from build123d import *

# Parameters (mm, degrees)
ESBO_O1_W                = 93
ESBO_O1_H                = 50
RESSALTO_EXTRUS_O1_DEPTH = 1.26
ESBO_O2_W                = 93
ESBO_O2_H                = 1.26
RESSALTO_EXTRUS_O2_DEPTH = 32.74
ESBO_O3_W                = 1.26
ESBO_O3_H                = 50
RESSALTO_EXTRUS_O4_DEPTH = 32.74
RESSALTO_EXTRUS_O5_START = 25
RESSALTO_EXTRUS_O5_DEPTH = 67
FILETE1_R                = 1
FILETE2_R                = 1
ESBO_O6_W                = 1.26
ESBO_O6_H                = 50
RESSALTO_EXTRUS_O6_DEPTH = 31.48
ESBO_O7_W                = 11
ESBO_O7_H                = 2.5
CORTE_EXTRUS_O1_DEPTH    = 1.26
ESBO_O8_W                = 13
ESBO_O8_H                = 2.5
CORTE_EXTRUS_O2_DEPTH    = 1.26
RESSALTO_EXTRUS_O7_DEPTH = 2
RESSALTO_EXTRUS_O8_DEPTH = 2
ESBO_O13_R               = 0.5
RESSALTO_EXTRUS_O9_DEPTH = 4


with BuildPart() as part:
    # Esboço1 → Ressalto-extrusão1 (new body)
    with BuildSketch(Plane(origin=(0, 0, 0), x_dir=(1, 0, 0), z_dir=(0, 1, 0))):
        with Locations((46.5, -25)):
            Rectangle(ESBO_O1_W, ESBO_O1_H)
    extrude(amount=RESSALTO_EXTRUS_O1_DEPTH)

    # Esboço2 → Ressalto-extrusão2 (add)
    with BuildSketch(Plane(origin=(0, 0, 0), x_dir=(1, 0, 0), z_dir=(0, 1, 0))):
        with Locations((46.5, -0.63)):
            Rectangle(ESBO_O2_W, ESBO_O2_H)
        with Locations((46.5, -49.37)):
            Rectangle(ESBO_O2_W, ESBO_O2_H)
    extrude(amount=RESSALTO_EXTRUS_O2_DEPTH)

    # Esboço3 → Ressalto-extrusão4 (add)
    with BuildSketch(Plane(origin=(0, 0, 0), x_dir=(1, 0, 0), z_dir=(0, 1, 0))):
        with Locations((92.37, -25)):
            Rectangle(ESBO_O3_W, ESBO_O3_H)
    extrude(amount=RESSALTO_EXTRUS_O4_DEPTH)

    # Esboço5 → Ressalto-extrusão5 (add)
    with BuildSketch(Plane(origin=(0, 0, 0), x_dir=(0, 0, -1), z_dir=(1, 0, 0)).offset(RESSALTO_EXTRUS_O5_START)):
        Polygon((0, 32.74), (-3.26, 32.74), (0, 29.48), align=None)
        Polygon((-50, 32.74), (-46.74, 32.74), (-50, 29.48), align=None)
    extrude(amount=RESSALTO_EXTRUS_O5_DEPTH)

    # Filete1
    filete1_edges = [part.edges().sort_by_distance(p)[0] for p in [
        (25, 31.74, 47.74),
    ]]
    fillet(filete1_edges, radius=FILETE1_R)

    # Filete2
    filete2_edges = [part.edges().sort_by_distance(p)[0] for p in [
        (25, 31.74, 2.26),
    ]]
    fillet(filete2_edges, radius=FILETE2_R)

    # Esboço6 → Ressalto-extrusão6 (add)
    with BuildSketch(Plane(origin=(0, 0, 0), x_dir=(1, 0, 0), z_dir=(0, 1, 0))):
        with Locations((0.63, -25)):
            Rectangle(ESBO_O6_W, ESBO_O6_H)
    extrude(amount=RESSALTO_EXTRUS_O6_DEPTH)

    # Esboço7 → Corte-extrusão1 (cut)
    with BuildSketch(Plane.ZY):
        with Locations((25, 2.51)):
            Rectangle(ESBO_O7_W, ESBO_O7_H)
    extrude(amount=-CORTE_EXTRUS_O1_DEPTH, mode=Mode.SUBTRACT)

    # Esboço8 → Corte-extrusão2 (cut)
    with BuildSketch(Plane(origin=(93, 0, 0), x_dir=(0, 0, -1), z_dir=(1, 0, 0))):
        with Locations((-25, 2.51)):
            Rectangle(ESBO_O8_W, ESBO_O8_H)
    extrude(amount=-CORTE_EXTRUS_O2_DEPTH, mode=Mode.SUBTRACT)

    # Esboço10 → Ressalto-extrusão7 (add)
    with BuildSketch(Plane(origin=(0, 1.26, 0), x_dir=(1, 0, 0), z_dir=(0, 1, 0))):
        Polygon((4, -14), (4, -17), (8, -17), (8, -19), (10.1, -19), (10.1, -14), align=None)
        Polygon((4, -33), (4, -36), (10.1, -36), (10.1, -31), (8, -31), (8, -33), align=None)
    extrude(amount=RESSALTO_EXTRUS_O7_DEPTH)

    # Esboço11 → Ressalto-extrusão8 (add)
    with BuildSketch(Plane(origin=(0, 1.26, 0), x_dir=(1, 0, 0), z_dir=(0, 1, 0))):
        Polygon((87.74, -12.74), (82.9, -12.74), (82.9, -18), (85, -18), (85, -16), (87.74, -16), align=None)
        Polygon((87.74, -34), (87.74, -37.26), (82.9, -37.26), (82.9, -32), (85, -32), (85, -34), align=None)
    extrude(amount=RESSALTO_EXTRUS_O8_DEPTH)

    # Esboço13 → Ressalto-extrusão9 (add)
    with BuildSketch(Plane.XZ):
        with Locations(Location((92.37, 30.775, 0), (0, 0, 90))):
            Circle(ESBO_O13_R)
        with Locations(Location((92.37, 29.175, 0), (0, 0, 90))):
            Circle(ESBO_O13_R)
        with Locations(Location((92.37, 27.575, 0), (0, 0, 90))):
            Circle(ESBO_O13_R)
        with Locations(Location((92.37, 25.975, 0), (0, 0, 90))):
            Circle(ESBO_O13_R)
        with Locations(Location((92.37, 24.025, 0), (0, 0, 90))):
            Circle(ESBO_O13_R)
        with Locations(Location((92.37, 22.425, 0), (0, 0, 90))):
            Circle(ESBO_O13_R)
        with Locations(Location((92.37, 20.825, 0), (0, 0, 90))):
            Circle(ESBO_O13_R)
        with Locations(Location((92.37, 19.225, 0), (0, 0, 90))):
            Circle(ESBO_O13_R)
        with Locations((0.63, 19.225)):
            Circle(ESBO_O13_R)
        with Locations(Location((0.63, 20.825, 0), (0, 0, 90))):
            Circle(ESBO_O13_R)
        with Locations(Location((0.63, 22.425, 0), (0, 0, 90))):
            Circle(ESBO_O13_R)
        with Locations(Location((0.63, 24.025, 0), (0, 0, 90))):
            Circle(ESBO_O13_R)
        with Locations(Location((0.63, 25.975, 0), (0, 0, 90))):
            Circle(ESBO_O13_R)
        with Locations(Location((0.63, 27.575, 0), (0, 0, 90))):
            Circle(ESBO_O13_R)
        with Locations(Location((0.63, 29.175, 0), (0, 0, 90))):
            Circle(ESBO_O13_R)
        with Locations((0.63, 30.775)):
            Circle(ESBO_O13_R)
    extrude(amount=-RESSALTO_EXTRUS_O9_DEPTH)


solid = part.part
CAD build for the part. Positions are in the model's coordinates, mm. A direction names the side the tool comes from. Round coordinates to 2 decimals unless told otherwise and drop trailing zeros. Order: outer loops, then holes, each group sorted by start corner. A loop starts at its lowest first (then second) coordinate and runs counter-clockwise, first axis right, second up. Notation, with made-up numbers: (-13.75, 35) -> (11.25, 35) arc R24 ccw to (11.25, 59) -> close; hole circle Ø1 at (44.25, 27). An arc over 180 degrees is marked (long way). Write item = value, one per line. Start each with the question number.
(1) Pull direction Z, two halves, no side cores. Call faces 1 (the flat face through (46, 16, 50)), 2 (the flat face through (0, 16, 25)), 3 (the flat face through (10.1, 2, 34)): released by +Z, released by -Z, zero draft, split by the parting line, or undercut.
(2) Probe line 1 (Z direction, x = 25, y = 18.5); line 2 (X direction, y = 12.5, z = 11); line 3 (Y direction, x = 40, z = 11.5). List the from-to ranges inside material, lowest first. Write a range as [from, to].
(3) Pin check, flat tip, straight feed: P1, Ø2.5, axis at x = 84.5, z = 15.5, coming from the +Y side. Stop position of the tip, or through.
(4) Cut at A-A, the plane z = 39.5. List the corners of the cut face in (x, y), then the cut area to 3 significant figures.
(5) Which spindle directions (+Z, -Z, +X, -X, +Y, -Y) get a long thin tool onto all of the face, cutting with end or side? Do faces 4 (the flat face through (58.41, 31.75, 2.27)), 5 (the flat face through (93, 16, 25)), 6 (the flat face through (87.74, 2, 36)). Say none if no direction does.
(6) Cut at C-C, the plane y = 29. List the corners of the cut face in (x, z), then the cut area to 3 significant figures.
(7) Cut at B-B, the plane x = 42.5. List the corners of the cut face in (y, z).
Model answer:
q1.face_1 = released by +Z
q1.face_2 = zero draft
q1.face_3 = undercut
q2.line_1 = [0, 1.26], [48.74, 50]
q2.line_2 = [0, 1.26], [91.74, 93]
q2.line_3 = [0, 1.26]
q3.P1 = 3.26
q4.outline = (0, 0) -> (93, 0) -> (93, 32.74) -> (91.74, 32.74) -> (91.74, 1.26) -> (1.26, 1.26) -> (1.26, 31.48) -> (0, 31.48) -> close
q4.area = 195 mm2
q5.face_4 = none
q5.face_5 = +Z, -Z, +X, +Y, -Y
q5.face_6 = +Y
q6.outline = (0, 0) -> (93, 0) -> (93, 50) -> (0, 50) -> close; hole (1.26, 1.26) -> (91.74, 1.26) -> (91.74, 48.74) -> (1.26, 48.74) -> close
q6.area = 354 mm2
q7.outline = (0, 0) -> (32.74, 0) -> (32.74, 3.26) -> (30.74, 1.26) -> (1.26, 1.26) -> (1.26, 48.74) -> (30.74, 48.74) -> (32.74, 46.74) -> (32.74, 50) -> (0, 50) -> close
